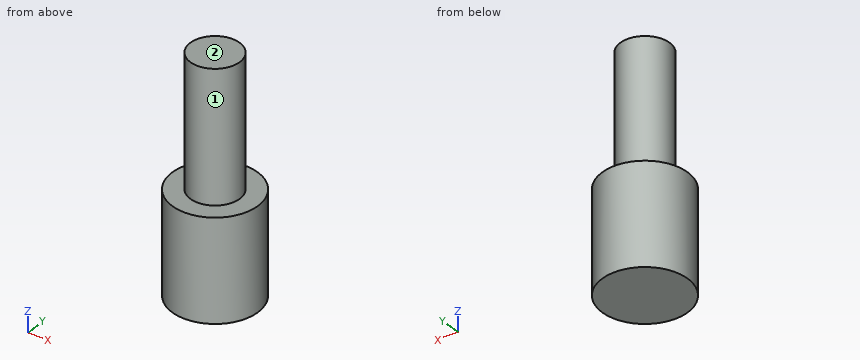
```python
from build123d import *

# Parameters (mm, degrees)
CYLINDER_R        = 2.95
CYLINDER_DEPTH    = 7
CYLINDER001_R     = 1.7
CYLINDER001_DEPTH = 10


with BuildPart() as m3bolthead:
    # Cylinder → Cylinder (new body)
    with BuildSketch(Plane.XY):
        Circle(CYLINDER_R)
    extrude(amount=CYLINDER_DEPTH)


with BuildPart() as m3bolt:
    # Cylinder001 → Cylinder001 (new body)
    with BuildSketch(Plane.XY.offset(6)):
        Circle(CYLINDER001_R)
    extrude(amount=CYLINDER001_DEPTH)

    # Fusion: union M3BoltHead
    add(m3bolthead.part)


solid = m3bolt.part
```
Here's how the part is built. I have some questions about the finished solid (model axes, mm). Face numbers are marked on the shaded views. A direction names the side the tool comes from. Give positions to 0.01 mm unless a question says otherwise; leave off trailing zeros. Loops run counter-clockwise (first coordinate to the right, second up) from the corner with the lowest first, then second, coordinate; pieces in that order, holes last. Notation, with made-up numbers: M 39,29 L 63,29 A19 cw 63,38 Z; hole C 50.25,22.5 d5. An arc over 180 degrees is marked long. Return JSON: item names as keys, results as strings.
Item 1: I'm going to push flat-ended pins straight in: pin 1 Ø3 at (x, z) = (2, 7.5) entering from -Y; pin 2 Ø1.5 at (y, z) = (-1.5, 10) entering from +X; pin 3 Ø3 at (x, z) = (-1.5, 14) entering from -Y. Where does each tip first touch, or does it pass through?
A:
{"pin 1": "stops at y = -2.89", "pin 2": "stops at x = 1.53", "pin 3": "stops at y = -1.7"}
Item 2: Please list where these lines run through material, in increasing order: line 1 (Z direction, x = 0.6, y = -1.7); line 2 (Y direction, x = -0.05, z = 10.5).
A:
{"line 1": "z = 0 to 7", "line 2": "y = -1.7 to 1.7"}
Item 3: On a 3-axis mill with a long thin cutter (end or side, diameter ignored), from which of +Z, -Z, +X, -X, +Y, -Y can I reach the whole of each face in a straight line? I mean the marked faces 1 and 2. Say none if no direction works.
A:
{"face 1": "+Z", "face 2": "+Z, +X, -X, +Y, -Y"}
Item 4: Imagine slicing it at C-C on z = 5.25. List the corners of the cut face in (x, y) for me.
A:
{"outline": "C 0,0 d5.9"}
Item 5: Imagine slicing it at D-D on z = 15. List the corners of the cut face in (x, y) for me.
A:
{"outline": "C 0,0 d3.4"}
Item 6: Imagine slicing it at A-A on y = 0. List the corners of the cut face in (x, z) for me, then the cut area to 3 significant figures.
A:
{"outline": "M -2.95,0 L 2.95,0 L 2.95,7 L 1.7,7 L 1.7,16 L -1.7,16 L -1.7,7 L -2.95,7 Z", "area": "71.9 mm^2"}
